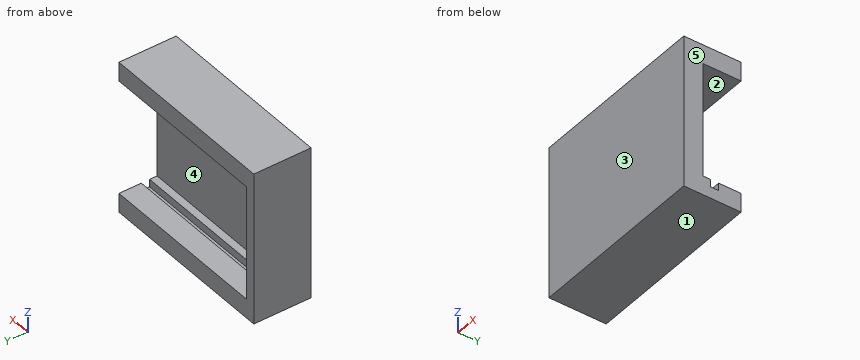
```python
from build123d import *

# Parameters (mm, degrees)
F1_DEPTH = 203.2
F0_W     = 228.6
F0_H     = 10
F2_DEPTH = 25.4
F0_H_2   = 29.8
F0_H_3   = 11
F3_DEPTH = 15.24
F4_W     = 228.6
F4_H     = 50.8
F5_DEPTH = 25.4
F6_W     = 33.1639014184
F6_H     = 23.3497917652
F7_DEPTH = 25.4
F8_W     = 231.14
F8_H     = 60.0164352887
F9_DEPTH = 0.254


# Not quite as in the source:
# - a feature names something its author has since deleted; it is built from what else it names


with BuildPart() as f1:
    # F0 (on Top) → F1 (new body)
    with BuildSketch(Plane.XY):
        Polygon((-143.864646554, -49.5614223182), (97.435353446, -49.5614223182), (97.435353446, -24.1614223182), (-131.164646554, -24.1614223182), (-131.164646554, -14.1614223182), (-131.164646554, -3.1614223182), (-131.164646554, 26.6385776818), (-143.864646554, 26.6385776818), align=None)
    extrude(amount=F1_DEPTH)

    # F4 (on face) → F5 (join)
    with BuildSketch(Plane.XY.offset(203.2)):
        with Locations((-16.864646554, 1.2385776818)):
            Rectangle(F4_W, F4_H)
    extrude(amount=-F5_DEPTH)



with BuildPart() as f2:
    # F0 (on Top) → F2 (new body)
    with BuildSketch(Plane.XY):
        with Locations((-16.864646554, -19.1614223182)):
            Rectangle(F0_W, F0_H)
    extrude(amount=F2_DEPTH)


with BuildPart() as f2b:
    # F0 (on Top) → F2, piece 2 (new body)
    with BuildSketch(Plane.XY):
        with Locations((-16.864646554, 11.7385776818)):
            Rectangle(F0_W, F0_H_2)
    extrude(amount=F2_DEPTH)


with BuildPart() as f3:
    # F0 (on Top) → F3 (new body)
    with BuildSketch(Plane.XY):
        with Locations((-16.864646554, -8.6614223182)):
            Rectangle(F0_W, F0_H_3)
    extrude(amount=F3_DEPTH)


with BuildPart() as f1_1:
    add(f1.part)

    add(f2.part)  # F7 merges F2
    # F6 (on face) → F7 (join)
    with BuildSketch(Plane.YZ.offset(97.435353446)):
        with Locations((-32.979471609, 11.6748958826)):
            Rectangle(F6_W, F6_H)
    extrude(amount=-F7_DEPTH)


    add(f2b.part)  # F9 merges F2b

    add(f3.part)  # F9 merges F3
    # F8 (on face) → F9 (join)
    with BuildSketch(Plane(origin=(0, 0, 0), x_dir=(1, 0, 0), z_dir=(0, 0, -1))):
        with Locations((-18.134646554, 3.3696399626)):
            Rectangle(F8_W, F8_H)
    extrude(amount=-F9_DEPTH)


solid = f1_1.part
```
Read the model definition and answer for the solid it produces. Units are mm, in the model's axes. Face numbers are marked on the shaded views. A direction names the side the tool comes from. Coordinates: 2 decimals unless noted, no trailing zeros. Write each loop counter-clockwise with the first axis right and the second up, starting at its lowest first coordinate (ties: lowest second). Pieces come first, ordered by that corner, then holes. Notation, with made-up numbers: (26.25, -4.75) -> (43.25, -4.75) arc R34 ccw to (43.25, 33.25) -> close; hole circle Ø9 at (-38.5, -14.75). An arc over 180 degrees is marked (long way). Answer as a JSON object with one key per item and string values.
Q1. The part is cut by section B-B on x = 47. Give the vertices of the cut face in (y, z).
The answers:
{"outline": "(-49.56, 0) -> (26.64, 0) -> (26.64, 25.4) -> (-3.16, 25.4) -> (-3.16, 15.24) -> (-14.16, 15.24) -> (-14.16, 25.4) -> (-24.16, 25.4) -> (-24.16, 177.8) -> (26.64, 177.8) -> (26.64, 203.2) -> (-49.56, 203.2) -> close"}
Q2. The part is cut by section A-A on y = -8. Give the vertices of the cut face in (x, z).
The answers:
{"outline": "(-143.86, 0) -> (97.44, 0) -> (97.44, 15.24) -> (-131.16, 15.24) -> (-131.16, 177.8) -> (97.44, 177.8) -> (97.44, 203.2) -> (-143.86, 203.2) -> close"}
Q3. A flat-ended cylindrical pin translates along its axis: pin 1 Ø2 at (x, z) = (54, 150) entering from +Y. Find the tip coordinate at first contact, or state that the pin passes through.
The answers:
{"pin 1": "stops at y = -24.16"}
Q4. The part is cut by section C-C on z = 56.5. Give the vertices of the cut face in (x, y).
The answers:
{"outline": "(-143.86, -49.56) -> (97.44, -49.56) -> (97.44, -24.16) -> (-131.16, -24.16) -> (-131.16, 26.64) -> (-143.86, 26.64) -> close"}
Q5. The part is cut by section D-D on y = 21. Give the vertices of the cut face in (x, z).
The answers:
{"outline": "(-143.86, 0) -> (97.44, 0) -> (97.44, 25.4) -> (-131.16, 25.4) -> (-131.16, 177.8) -> (97.44, 177.8) -> (97.44, 203.2) -> (-143.86, 203.2) -> close"}
Q6. Consider line 1 (Z direction, x = 65, y = -12); line 2 (Z direction, x = 54, y = 3); line 3 (Y direction, x = -67, z = 23). Determine where each line is inside the solid, lowest interval first. Write a range as [from, to].
The answers:
{"line 1": "z = [0, 15.24], [177.8, 203.2]", "line 2": "z = [0, 25.4], [177.8, 203.2]", "line 3": "y = [-49.56, -14.16], [-3.16, 26.64]"}
Q7. A tool of negligible diameter and unlimited length cuts with its end or side. For the marked faces 4 and 5, from which of +Z, -Z, +X, -X, +Y, -Y can it reach the whole face along a straight path? Write none if from no direction.
The answers:
{"face 4": "+X, +Y", "face 5": "+Z, -Z, +X, +Y, -Y"}
Q8. Determine the mould class of the marked faces 1, 2 and 3 for opening direction Z: pulls with the +Z half, pulls with the -Z half, needs draft (parallel to the pull), parting line crosses it, or undercut.
The answers:
{"face 1": "pulls with the -Z half", "face 2": "undercut", "face 3": "needs draft"}
